from build123d import *

# Parameters (mm, degrees)
SKETCH1_W           = 150
SKETCH1_H           = 30
BOSS_EXTRUDE1_DEPTH = 30
SKETCH2_R           = 10
BOSS_EXTRUDE2_DEPTH = 10
FILLET1_R           = 10
SKETCH3_W           = 40
SKETCH3_H           = 20
CUT_EXTRUDE1_DEPTH  = 27.8
SKETCH4_R           = 2.5
CUT_EXTRUDE2_DEPTH  = 27.8
CUT_EXTRUDE3_DEPTH  = 31
CHAMFER1_SIZE       = 3


with BuildPart() as part:
    # Sketch1 → Boss-Extrude1 (new body)
    with BuildSketch(Plane.XY):
        Rectangle(SKETCH1_W, SKETCH1_H)
    extrude(amount=BOSS_EXTRUDE1_DEPTH)

    # Sketch2 → Boss-Extrude2 (add)
    with BuildSketch(Plane.XY.offset(30)):
        with Locations((-55, 0)):
            Circle(SKETCH2_R)
    extrude(amount=BOSS_EXTRUDE2_DEPTH)

    # Fillet1
    fillet1_edges = [part.edges().sort_by_distance(p)[0] for p in [
        (75, -15, 15),
        (-75, -15, 15),
        (-75, 15, 15),
        (75, 15, 15),
    ]]
    fillet(fillet1_edges, radius=FILLET1_R)

    # Sketch3 → Cut-Extrude1 (cut)
    with BuildSketch(Plane(origin=(0, 0, 0), x_dir=(-1, 0, 0), z_dir=(0, 0, -1))):
        with Locations((-45, 0)):
            Rectangle(SKETCH3_W, SKETCH3_H)
    extrude(amount=-CUT_EXTRUDE1_DEPTH, mode=Mode.SUBTRACT)

    # Sketch4 → Cut-Extrude2 (cut)
    with BuildSketch(Plane(origin=(0, 0, 27.8), x_dir=(-1, 0, 0), z_dir=(0, 0, -1))):
        with Locations((-55, 0)):
            Circle(SKETCH4_R)
    extrude(amount=-CUT_EXTRUDE2_DEPTH, mode=Mode.SUBTRACT)

    # Sketch5 → Cut-Extrude3 (cut, through all)
    with BuildSketch(Plane(origin=(0, 15, 0), x_dir=(1, 0, 0), z_dir=(0, 1, 0))):
        Polygon((-60, -7.5), (-60, -22.5), (-45.857864376, -17.5), (45.857864376, -17.5), (60, -22.5), (60, -7.5), (45.857864376, -12.5), (-45.857864376, -12.5), align=None)
    extrude(amount=-CUT_EXTRUDE3_DEPTH, mode=Mode.SUBTRACT)

    # Chamfer1
    chamfer1_edges = [part.edges().sort_by_distance(p)[0] for p in [
        (75, 0, 0),
        (75, 0, 30),
        (0, -15, 0),
        (-75, 0, 0),
        (0, 15, 0),
        (-72.071067812, 12.071067812, 0),
        (-72.071067812, -12.071067812, 0),
        (72.071067812, 12.071067812, 0),
        (72.071067812, -12.071067812, 0),
        (0, -15, 30),
        (0, 15, 30),
        (-75, 0, 30),
        (-72.071067812, 12.071067812, 30),
        (-72.071067812, -12.071067812, 30),
        (72.071067812, 12.071067812, 30),
        (72.071067812, -12.071067812, 30),
    ]]
    chamfer(chamfer1_edges, length=CHAMFER1_SIZE)


solid = part.part
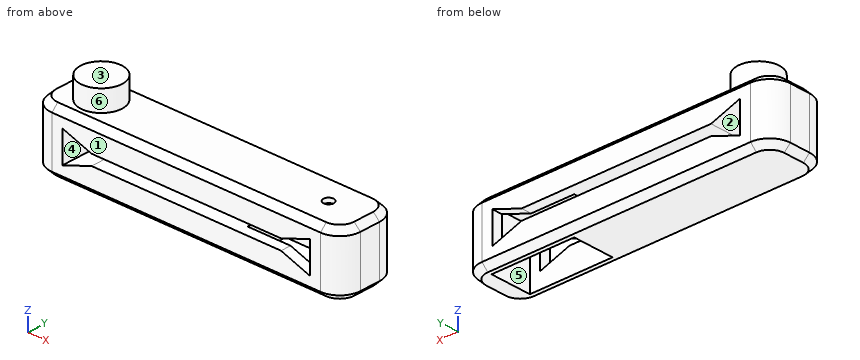
CAD build for the part. Positions are in the model's coordinates, mm. Face numbers are marked on the shaded views. A direction names the side the tool comes from. Give positions to 0.01 mm unless a question says otherwise; leave off trailing zeros. Loops run counter-clockwise (first coordinate to the right, second up) from the corner with the lowest first, then second, coordinate; pieces in that order, holes last. Notation, with made-up numbers: M -11.75,-1 L -1.75,-1 A20 cw -1.75,32 Z; hole C 2,48 d1. An arc over 180 degrees is marked long. Answer in a Markdown table with one row per item. Add a question column.
Item 1: Drop flat-ended pins along their axis: P1, Ø8, axis at x = -37.5, z = 31.5, coming from the +Y side; P2, Ø16, axis at x = 43, y = -1.5, coming from the -Z side; P3, Ø6, axis at x = -24, z = 16.5, coming from the -Y side; P4, Ø9, axis at x = 0.5, y = 0.5, coming from the +Z side. Give the stop position or say it passes through.
Item 2: Probe probe 1 along Z at (x, y) = (-20.5, -11); probe 2 along Y at (x, z) = (60.5, 12); probe 3 along X at (y, z) = (2, 25). List the from-to ranges inside material, lowest first.
Item 3: Band-saw the part on A-A on x = 55. Give the cut face in (y, z), then the cut area to 3 significant figures.
Item 4: Tool access for the marked faces 4, 5 and 6: list every direction of +Z, -Z, +X, -X, +Y, -Y with a clear straight run to the whole face (end or side of a thin tool).
Item 5: Band-saw the part on D-D on z = 9.5. Give the cut face in (x, y), then the cut area to 3 significant figures.
Item 6: Band-saw the part on C-C on x = 39. Give the cut face in (y, z).
Item 7: Mould opens along Z. For the marked faces 1, 2 and 3 say: +Z half, -Z half, draft (parallel to the pull), parting line (faces both ways), or undercut.
Item 8: Band-saw the part on B-B on y = 0. Give the cut face in (x, z), then the cut area to 3 significant figures.
Reply:
| question | item | result |
|---|---|---|
| 1 | P1 | stops at y = 14.5 |
| 1 | P2 | stops at z = 27.8 |
| 1 | P3 | stops at y = -15 |
| 1 | P4 | stops at z = 30 |
| 2 | probe 1 | z = 0 to 12.5, 17.5 to 30 |
| 2 | probe 2 | y = -15 to -10, 10 to 15 |
| 2 | probe 3 | x = -75 to 25, 65 to 75 |
| 3 | outline | M -15,3 L -12,0 L -10,0 L -10,9.27 L -15,9.27 Z; M -15,20.73 L -10,20.73 L -10,27.8 L -2.5,27.8 L -2.5,30 L -12,30 L -15,27 Z; M 2.5,27.8 L 10,27.8 L 10,20.73 L 15,20.73 L 15,27 L 12,30 L 2.5,30 Z; M 10,0 L 12,0 L 15,3 L 15,9.27 L 10,9.27 Z |
| 3 | area | 200 mm^2 |
| 4 | face 4 | +Y, -Y |
| 4 | face 5 | -Z |
| 4 | face 6 | +Z |
| 5 | outline | M -75,-5 A10 ccw -65,-15 L -60,-15 L -60,15 L -65,15 A10 ccw -75,5 Z; M -54.34,-15 L 54.34,-15 L 54.34,-10 L 25,-10 L 25,10 L 54.34,10 L 54.34,15 L -54.34,15 Z; M 60,-15 L 65,-15 A10 ccw 75,-5 L 75,5 A10 ccw 65,15 L 60,15 L 60,10 L 65,10 L 65,-10 L 60,-10 Z |
| 5 | area | 3,390 mm^2 |
| 6 | outline | M -15,3 L -12,0 L -10,0 L -10,12.5 L -15,12.5 Z; M -15,17.5 L -10,17.5 L -10,27.8 L 10,27.8 L 10,17.5 L 15,17.5 L 15,27 L 12,30 L -12,30 L -15,27 Z; M 10,0 L 12,0 L 15,3 L 15,12.5 L 10,12.5 Z |
| 7 | face 1 | draft |
| 7 | face 2 | undercut |
| 7 | face 3 | +Z half |
| 8 | outline | M -75,3 L -72,0 L 25,0 L 25,12.5 L -45.86,12.5 L -60,7.5 L -60,22.5 L -45.86,17.5 L 25,17.5 L 25,27.8 L 52.5,27.8 L 52.5,30 L -45,30 L -45,40 L -65,40 L -65,30 L -72,30 L -75,27 Z; M 57.5,27.8 L 65,27.8 L 65,0 L 72,0 L 75,3 L 75,27 L 72,30 L 57.5,30 Z |
| 8 | area | 3,060 mm^2 |
